For this review, use the dimensioned drawing (mm, ordinates from the lowest corner) and the shaded views. Round coordinates to 2 decimals unless told otherwise and drop trailing zeros. Write each loop counter-clockwise with the first axis right and the second up, starting at its lowest first coordinate (ties: lowest second). Pieces come first, ordered by that corner, then holes. Notation, with made-up numbers: M 53,57 L 110,57 A36 cw 110,91 Z; hole C 19.25,-30 d4. An arc over 180 degrees is marked long. Use one line per item in the form item = value. Start each with the question number.
Item 1: For line 1 (X direction, y = 0.95, z = 65.9); line 2 (Z direction, x = 88.65, y = 0.6); line 3 (X direction, y = 0.25, z = 63.5), list the stretches that pass through material, from the lowest coordinate up. Write a range as [from, to].
Item 2: For P1, Ø1, axis at y = 1, z = 68.5, coming from the -X side, flat-tipped, find the tip position at first contact; note if it passes through.
Item 3: Add section A-A (z = 68.5). State the section outline as (x, y) points.
Item 4: Add section B-B (x = 62.65). State the section outline as (y, z) points.
Item 5: Add section C-C (y = 0.75). State the section outline as (x, z) points, and give its area (3 significant figures).
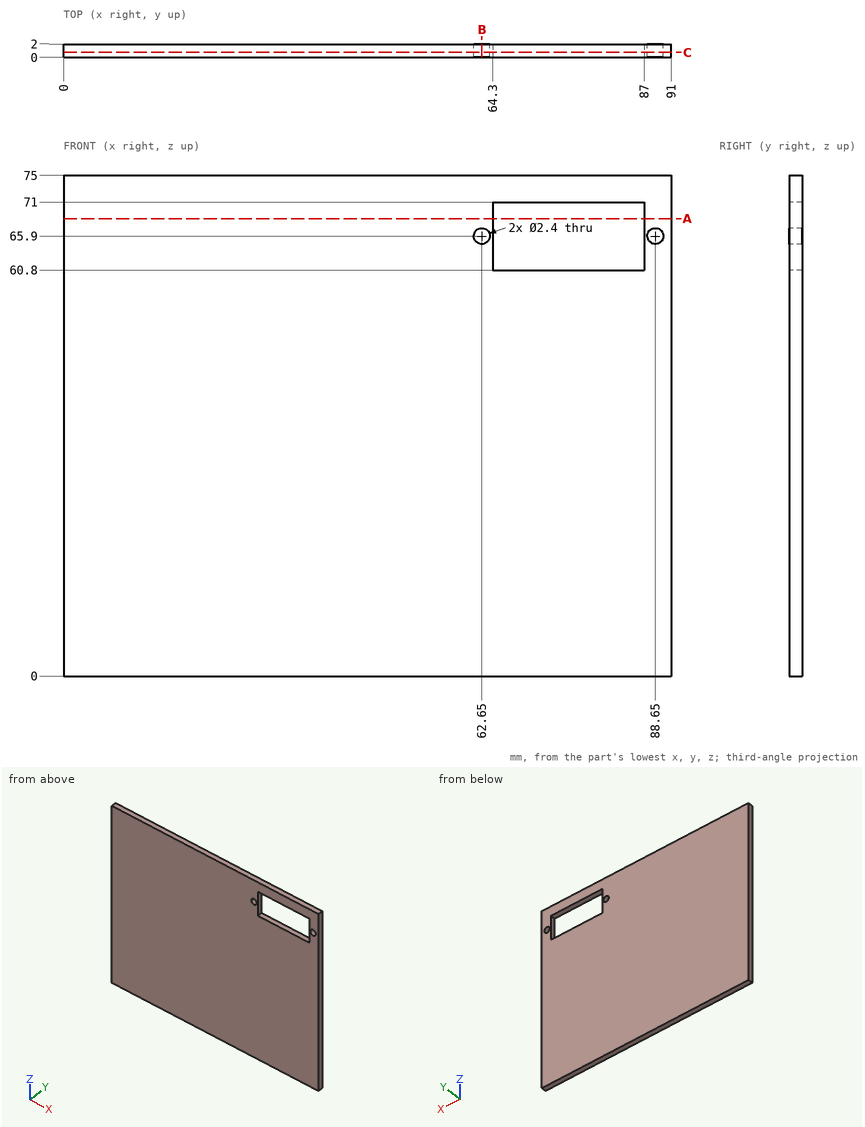
Calculated:
q1.line_1 = [0, 61.45], [63.85, 64.3], [87, 87.45], [89.85, 91]
q1.line_2 = [0, 64.7], [67.1, 75]
q1.line_3 = [0, 64.3], [87, 91]
q2.P1 = 0
q3.outline = M 0,0 L 64.3,0 L 64.3,2 L 0,2 Z; M 87,0 L 91,0 L 91,2 L 87,2 Z
q4.outline = M 0,0 L 2,0 L 2,64.7 L 0,64.7 Z; M 0,67.1 L 2,67.1 L 2,75 L 0,75 Z
q5.outline = M 0,0 L 91,0 L 91,75 L 0,75 Z; hole C 62.65,65.9 d2.4; hole M 64.3,60.8 L 87,60.8 L 87,71 L 64.3,71 Z; hole C 88.65,65.9 d2.4
q5.area = 6,580 mm^2
